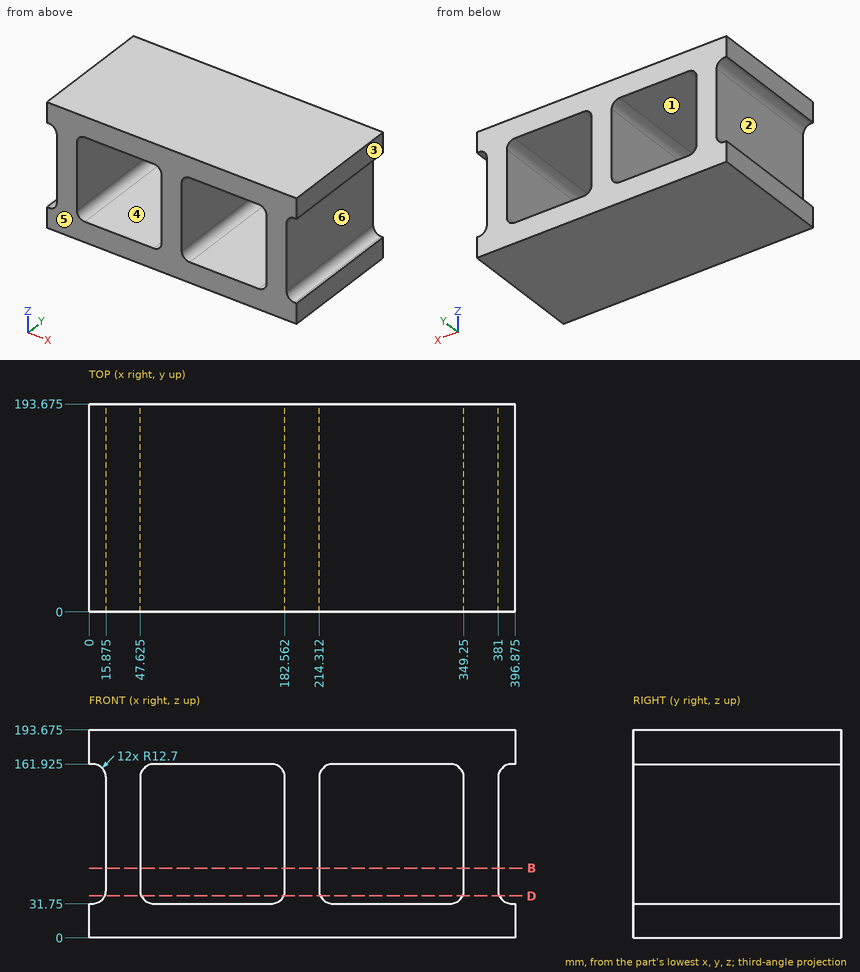
Drawing for the job (mm, zero at the part's lowest x, y, z). A direction names the side the tool comes from. Coordinates: 2 decimals unless noted, no trailing zeros. Write each loop counter-clockwise with the first axis right and the second up, starting at its lowest first coordinate (ties: lowest second). Pieces come first, ordered by that corner, then holes. Notation, with made-up numbers: (36.25, 75.25) -> (87.25, 75.25) arc R24 ccw to (87.25, 98.25) -> close; hole circle Ø10 at (48, 9). An arc over 180 degrees is marked (long way). One line per item, written item: value. Start each with the question number.
1) Slice it at B-B on z = 65. Count the separate pieces of the cut face and the enclosed holes in it, then the cut area to 3 significant figures.
2) Pull direction X, two halves, no side cores. Call the marked faces 1, 2 and 3: +X half, -X half, draft (parallel to the pull), parting line (faces both ways), or undercut.
3) Probe probe 1 along X at (y, z) = (117.5, 34) (1 decimal); probe 2 along Z at (x, y) = (177.5, 82.5) (1 decimal); probe 3 along Z at (x, y) = (58, 33) (1 decimal). List the from-to ranges inside material, lowest first.
4) Flat gauge pins, fed straight in: pin 1 Ø1 at (x, y) = (206.5, 144) entering from -Z; pin 2 Ø1 at (y, z) = (30, 99) entering from -X (1 decimal). Where does each tip first touch, or does it go through?
5) Slice it at D-D on z = 39. Write the cut outline in (x, y) (1 decimal).
6) Which spindle directions (+Z, -Z, +X, -X, +Y, -Y) get a long thin tool onto all of the face, cutting with end or side? Do the marked faces 4, 5 and 6. Say none if no direction does.
Answers follow:
1. separate pieces: 3
1. enclosed holes: 0
1. area: 18,400 mm2
2. face 1: undercut
2. face 2: -X half
2. face 3: +X half
3. probe 1: 10.4 to 53.1, 177.1 to 219.8, 343.8 to 386.5
3. probe 2: 0 to 34.3, 159.4 to 193.7
3. probe 3: 0 to 32, 161.7 to 193.7
4. pin 1: z = 0
4. pin 2: x = 15.9
5. outline: (14.6, 0) -> (48.9, 0) -> (48.9, 193.7) -> (14.6, 193.7) -> close; (181.3, 0) -> (215.5, 0) -> (215.5, 193.7) -> (181.3, 193.7) -> close; (348, 0) -> (382.2, 0) -> (382.2, 193.7) -> (348, 193.7) -> close
6. face 4: +Y, -Y
6. face 5: +Z, -Z, +X, -X, -Y
6. face 6: +X, +Y, -Y
